The model under review builds one solid part; all positions refer to its coordinate system, in mm. A direction names the side the tool comes from. Coordinates: 2 decimals unless noted, no trailing zeros. Order: outer loops, then holes, each group sorted by start corner. A loop starts at its lowest first (then second) coordinate and runs counter-clockwise, first axis right, second up.
```python
from build123d import *

# Parameters (mm, degrees)
EXTRUDE_1_DEPTH = 1.5
SKETCH_2_R      = 3.5
EXTRUDE_2_DEPTH = 1.5
SKETCH_3_R      = 2.5
EXTRUDE_3_DEPTH = 3


with BuildPart() as part:
    # 草图1 → 凸台-拉伸1 (new body)
    with BuildSketch(Plane(origin=(0, 0, 0), x_dir=(1, 0, 0), z_dir=(0, 1, 0))):
        with BuildLine():
            Line((0, 5), (12, 5))
            ThreePointArc((12, 5), (17, 0), (12, -5))
            Line((12, -5), (0, -5))
            ThreePointArc((0, -5), (-5, 0), (0, 5))
        make_face()
    extrude(amount=EXTRUDE_1_DEPTH)

    # 草图2 → 凸台-拉伸2 (add)
    with BuildSketch(Plane.XZ):
        with Locations(Location((12, 0, 0), (0, 0, 90))):
            Circle(SKETCH_2_R)
    extrude(amount=EXTRUDE_2_DEPTH)

    # 草图3 → 凸台-拉伸3 (add)
    with BuildSketch(Plane(origin=(0, 1.5, 0), x_dir=(1, 0, 0), z_dir=(0, 1, 0))):
        with Locations(Location((0, 0, 0), (0, 0, 270))):
            Circle(SKETCH_3_R)
    extrude(amount=EXTRUDE_3_DEPTH)


solid = part.part
```
(1) We need section D-D, the plane z = -2.25. Write out the cut boundary in (x, y).
A:
outline: (-4.47, 0) - (9.32, 0) - (9.32, -1.5) - (14.68, -1.5) - (14.68, 0) - (16.47, 0) - (16.47, 1.5) - (1.09, 1.5) - (1.09, 4.5) - (-1.09, 4.5) - (-1.09, 1.5) - (-4.47, 1.5) - close
(2) For pin 1 Ø5 at (x, z) = (6.5, 2) entering from +Y; pin 2 Ø3 at (x, y) = (-1.5, -1) entering from +Z; pin 3 Ø2 at (y, z) = (0.5, -1.5) entering from -X, all flat-tipped, find the tip position at first contact; note any pin that passes through.
A:
pin 1: stops at y = 1.5
pin 2: stops at z = 4.99
pin 3: stops at x = -4.97
(3) We need section C-C, the plane x = 3.5. Write out the cut boundary in (y, z).
A:
outline: (0, -5) - (1.5, -5) - (1.5, 5) - (0, 5) - close
(4) Machinability: for faces 1 (the face through (-5, 1, 0)), 2 (the face through (15.417, -0.74, -0.759)), 3 (the face through (-2.44, 2.98, -0.54)), which of the approach directions +Z, -Z, +X, -X, +Y, -Y give a long, thin tool a straight path to every point of the face, cutting with its end or side? Answer none if there is none.
A:
face 1: -X, +Y, -Y
face 2: -Y
face 3: +Y
(5) We need section A-A, the plane z = 0. Write out the cut boundary in (x, y), and give its area (3 significant figures).
A:
outline: (-5, 0) - (8.5, 0) - (8.5, -1.5) - (15.5, -1.5) - (15.5, 0) - (17, 0) - (17, 1.5) - (2.5, 1.5) - (2.5, 4.5) - (-2.5, 4.5) - (-2.5, 1.5) - (-5, 1.5) - close
area: 58.5 mm2
(6) Wall thickness on probe 1 along X at (y, z) = (-1.15, 0); probe 2 along Y at (x, z) = (8.75, -0.25); probe 3 along Y at (x, z) = (3.5, -1.75): over which ranges is each line inside the solid? List them lowest first.
A:
probe 1: x = 8.5 to 15.5
probe 2: y = -1.5 to 1.5
probe 3: y = 0 to 1.5
(7) We need section B-B, the plane y = 3. Write out the cut boundary in (x, z).
A:
outline: circle Ø5 at (0, 0)
